```python
from build123d import *

# Parameters (mm, degrees)
F1_DEPTH  = 60
F2_DEPTH  = 58
F5_DEPTH  = 60
F11_DEPTH = 25
F12_R     = 15


with BuildPart() as f1:
    # F0 (on Top) → F1 (new body)
    with BuildSketch(Plane.XY):
        with BuildLine():
            ThreePointArc((11, -30), (9.2813061641, -17.0032513647), (4.2433809964, -4.9))
            Line((4.2433809964, -4.9), (3.2433809964, -4.9))
            ThreePointArc((3.2433809964, -4.9), (8.2813061641, -17.0032513647), (10, -30))
            Line((10, -30), (11, -30))
        make_face()
        with BuildLine():
            Line((1, 0), (0, 0))
            ThreePointArc((0, 0), (0.5058928967, -0.6866474002), (1, -1.3818239575))
            Line((1, -1.3818239575), (1, 0))
        make_face()
        with BuildLine():
            ThreePointArc((4.2433809964, -55.1), (9.2813061641, -42.9967486353), (11, -30))
            Line((11, -30), (10, -30))
            ThreePointArc((10, -30), (8.2813061641, -42.9967486353), (3.2433809964, -55.1))
            Line((3.2433809964, -55.1), (4.2433809964, -55.1))
        make_face()
        with BuildLine():
            ThreePointArc((1, -60), (2.6937359795, -57.5976879479), (4.2433809964, -55.1))
            Line((4.2433809964, -55.1), (3.2433809964, -55.1))
            ThreePointArc((3.2433809964, -55.1), (2.1584060549, -56.8824998634), (1, -58.6181760425))
            Line((1, -58.6181760425), (1, -60))
        make_face()
        with BuildLine():
            ThreePointArc((1, -58.6181760425), (0.5058928967, -59.3133525998), (0, -60))
            Line((0, -60), (1, -60))
            Line((1, -60), (1, -58.6181760425))
        make_face()
        with BuildLine():
            ThreePointArc((4.2433809964, -4.9), (2.6937359795, -2.4023120521), (1, 0))
            Line((1, 0), (1, -1.3818239575))
            ThreePointArc((1, -1.3818239575), (2.1584060549, -3.1175001366), (3.2433809964, -4.9))
            Line((3.2433809964, -4.9), (4.2433809964, -4.9))
        make_face()
    extrude(amount=F1_DEPTH)

    # F0 (on Top) → F2 (join)
    with BuildSketch(Plane.XY):
        with BuildLine():
            Line((60, -4.9), (4.2433809964, -4.9))
            ThreePointArc((4.2433809964, -4.9), (9.2813061641, -17.0032513647), (11, -30))
            Line((11, -30), (60, -30))
            Line((60, -30), (60, -4.9))
        make_face()
        with BuildLine():
            Line((60, -30), (11, -30))
            ThreePointArc((11, -30), (9.2813061641, -42.9967486353), (4.2433809964, -55.1))
            Line((4.2433809964, -55.1), (60, -55.1))
            Line((60, -55.1), (60, -30))
        make_face()
    extrude(amount=F2_DEPTH)

    # F4 (on face) → F5 (cut)
    with BuildSketch(Plane.XZ.offset(55.1)):
        Polygon((60, 58), (25, 58), (60, 23), align=None)
    extrude(amount=-F5_DEPTH, mode=Mode.SUBTRACT)

    # F10: sweep along a path in F9
    with BuildLine(Plane.XZ.offset(30)) as f10_path:
        ThreePointArc((0, 25.1), (23.0896284171, 27.7230233964), (42.4998142724, 40.5001857276))
    # F7 (on Right) → F10 (sweep, cut)
    with BuildSketch(Plane.YZ):
        with BuildLine():
            Line((-30, 25.1), (-30, 2.5))
            ThreePointArc((-30, 2.5), (-14.0193867452, 9.1193867452), (-7.4, 25.1))
            Line((-7.4, 25.1), (-30, 25.1))
        make_face()
        with BuildLine():
            ThreePointArc((-7.4, 25.1), (-45.9806132548, 41.0806132548), (-30, 2.5))
            Line((-30, 2.5), (-30, 25.1))
            Line((-30, 25.1), (-7.4, 25.1))
        make_face()
    sweep(path=f10_path.line, mode=Mode.SUBTRACT)

    # F11 (cut): a face of the model
    f11_faces = [f1.faces().sort_by_distance(p)[0] for p in [
        (34.7646818914, -30, 46.1719723121),
    ]]
    extrude(f11_faces, amount=-F11_DEPTH, mode=Mode.SUBTRACT)

    # F12
    f12_edges = [f1.edges().sort_by_distance(p)[0] for p in [
        (14.62169, -55.1, 58),
        (14.62169, -4.9, 58),
        (60, -55.1, 11.5),
        (60, -4.9, 11.5),
    ]]
    fillet(f12_edges, radius=F12_R)


solid = f1.part
```
Verification items for the finished model (mm, model axes). A direction names the side the tool comes from. Give positions to 0.01 mm unless a question says otherwise; leave off trailing zeros. Write each loop counter-clockwise with the first axis right and the second up, starting at its lowest first coordinate (ties: lowest second). Pieces come first, ordered by that corner, then holes. Notation, with made-up numbers: M -2.75,52.5 L 24.25,52.5 A10 ccw 24.25,60.5 Z; hole C -25.5,60 d6. An arc over 180 degrees is marked long. One line per question, with ' | ' between items.
1) Section check A-A on y = -56. Enter the section's corners in (x, z), plus the area to 3 significant figures.
Result:
outline: M 2.71,0 L 3.71,0 L 3.71,60 L 2.71,60 Z | area: 60.0 mm2
2) Mould release check, pull along Z, two halves, no side actions. Record for faces 4 (the flat face through (30, -30, 0)), 5 (the flat face through (25, -4.9, 21)), 6 (the flat face through (10.4, -29.9, 60)), 7 (the cylindrical face through (25.064, -29.503, 54.932)): released by +Z, released by -Z, zero draft, split by the parting line, or undercut.
Result:
face 4: released by -Z | face 5: zero draft | face 6: released by +Z | face 7: undercut
3) Set-up check for faces 1 (the cylindrical face through (18.4, -52.29, 51.74)), 2 (the cylindrical face through (17.9, -7.52, 51.47)), 3 (the flat face through (24, -55.1, 21)): record each of +Z, -Z, +X, -X, +Y, -Y from which the full face is reachable in a straight line by a thin tool's end or side.
Result:
face 1: +Z, +X, -Y | face 2: +Z, +X, +Y | face 3: +Z, -Z, +X, -Y
4) Thickness scan on line 1 along X through (y, z) = (-20.5, 14.5); line 2 along Y through (x, z) = (14.5, 11); line 3 along Y through (x, z) = (24.5, 50). Record the ranges inside material, lowest first. Write a range as [from, to].
Result:
line 1: x = [42.5, 60] | line 2: y = [-55.1, -47.44], [-12.56, -4.9] | line 3: y = [-53.37, -41.63], [-18.37, -6.63]
5) Gauge pin test, flat ends, axial feed: pin 1 Ø12 at (x, y) = (32, -45) entering from -Z; pin 2 Ø7.5 at (x, y) = (19.5, -29) entering from +Z; pin 3 Ø5 at (x, y) = (40.5, -28.5) entering from +Z; pin 4 Ø12 at (y, z) = (-14.5, 53.5) entering from -X. Record the tip position at first contact, or that the pin passes through.
Result:
pin 1: stops at z = 0 | pin 2: stops at z = 58 | pin 3: stops at z = 12.44 | pin 4: stops at x = 5.14
